```python
from build123d import *

# Parameters (mm, degrees)
F0_W          = 457.2
F0_H          = 254
F1_DEPTH      = 12.7
F3_R          = 15.875
F4_DEPTH      = 25.4
F4_DEPTH_BACK = 25.4
F6_DEPTH      = 127
F6_DEPTH_BACK = 127


with BuildPart() as f1:
    # F0 (on Front) → F1 (new body)
    with BuildSketch(Plane.XZ):
        with Locations((228.6, -127)):
            Rectangle(F0_W, F0_H)
    extrude(amount=F1_DEPTH)

    # F3 (on offset) → F4 (join, two sides)
    with BuildSketch(Plane.XY.offset(-127)) as f4_sk:
        with BuildLine():
            ThreePointArc((25.4, 25.4), (17.9605122421, 7.4394877579), (0, 0))
            Line((0, 0), (25.4, 0))
            Line((25.4, 0), (50.8, 0))
            Line((50.8, 0), (76.2, 0))
            Line((76.2, 0), (101.6, 0))
            ThreePointArc((101.6, 0), (83.6394877579, 7.4394877579), (76.2, 25.4))
            ThreePointArc((76.2, 25.4), (50.8, 50.8), (25.4, 25.4))
        make_face()
        with Locations((50.8, 25.4)):
            Circle(F3_R, mode=Mode.SUBTRACT)
        with BuildLine():
            Line((425.45, 0), (450.85, 0))
            ThreePointArc((450.85, 0), (432.8894877579, 7.4394877579), (425.45, 25.4))
            ThreePointArc((425.45, 25.4), (400.05, 50.8), (374.65, 25.4))
            ThreePointArc((374.65, 25.4), (367.2105122421, 7.4394877579), (349.25, 0))
            Line((349.25, 0), (374.65, 0))
            Line((374.65, 0), (400.05, 0))
            Line((400.05, 0), (425.45, 0))
        make_face()
        with Locations((400.05, 25.4)):
            Circle(F3_R, mode=Mode.SUBTRACT)
    extrude(amount=F4_DEPTH)
    extrude(f4_sk.sketch, amount=-F4_DEPTH_BACK)

    # F5 (on offset) → F6 (cut, two sides)
    with BuildSketch(Plane.XY.offset(-127)) as f6_sk:
        Polygon((25.4, -43.3393605053), (25.4, 0), (25.4, 52.3727163672), (-28.9033520967, 52.3727163672), (-28.9033520967, -43.3393605053), align=None)
        Polygon((425.45, 52.3727163672), (425.45, 0), (425.45, -43.3393605053), (479.7533520967, -43.3393605053), (479.7533520967, 52.3727163672), align=None)
    extrude(amount=-F6_DEPTH, mode=Mode.SUBTRACT)
    extrude(f6_sk.sketch, amount=F6_DEPTH_BACK, mode=Mode.SUBTRACT)


solid = f1.part
```
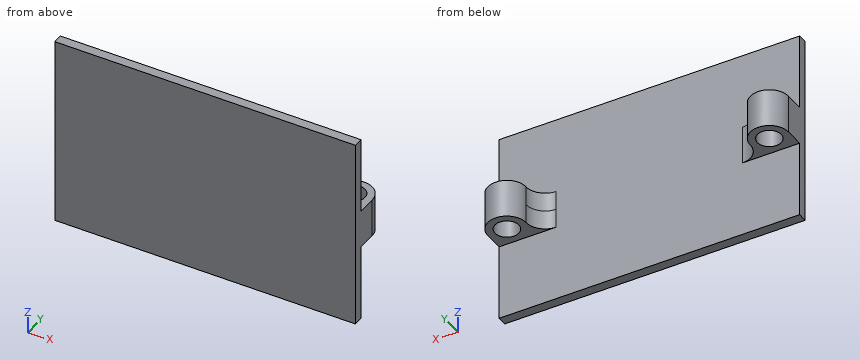
The listing builds one solid part. Answer for the finished solid, in the listing's coordinates (mm). Coordinates: 2 decimals unless noted, no trailing zeros. Loops run counter-clockwise (first coordinate to the right, second up) from the corner with the lowest first, then second, coordinate; pieces in that order, holes last. Notation, with made-up numbers: (80.5, 55.25) -> (121.5, 55.25) arc R10 cw to (121.5, 74.25) -> close; hole circle Ø6 at (44, 60.25). An arc over 180 degrees is marked (long way). Use one line per item in the form item = value. Start each with the question number.
Item 1: The part is cut by section B-B on z = -139.5. Determine the outline of the cut face in (x, y) (3 decimals), then the cut area to 3 significant figures.
Item 2: The part is cut by section D-D on x = 172. Determine the outline of the cut face in (y, z), then the cut area to 3 significant figures.
Item 3: The part is cut by section A-A on x = 400.05. Determine the outline of the cut face in (y, z) (3 decimals), then the cut area to 3 significant figures.
Item 4: The part is cut by section C-C on y = 5.5. Determine the outline of the cut face in (x, z).
Item 5: Flat-ended cylindrical pins translate along their axes: pin 1 Ø12 at (x, y) = (70.5, 27.5) entering from -Z; pin 2 Ø19 at (x, y) = (400.05, 25.4) entering from -Z (3 decimals). Find the tip coordinate at first contact, or state that the pin passes through.
Item 6: Consider L1, parallel to X at y = 25, z = -110; L2, parallel to Y at x = 50.8, z = -116 (3 decimals); L3, parallel to Y at x = 243.5, z = -191. Determine where each line is inside the solid, lowest interval first. Write a range as [from, to].
Answer key:
q1.outline = (25.4, -12.7) -> (425.45, -12.7) -> (425.45, 25.4) arc R25.4 ccw to (374.65, 25.4) arc R25.4 cw to (349.25, 0) -> (101.6, 0) arc R25.4 cw to (76.2, 25.4) arc R25.4 ccw to (25.4, 25.4) -> close; hole circle Ø31.75 at (50.8, 25.4); hole circle Ø31.75 at (400.05, 25.4)
q1.area = 8,380 mm2
q2.outline = (-12.7, -254) -> (0, -254) -> (0, 0) -> (-12.7, 0) -> close
q2.area = 3,230 mm2
q3.outline = (-12.7, -254) -> (0, -254) -> (0, -152.4) -> (9.525, -152.4) -> (9.525, -101.6) -> (0, -101.6) -> (0, 0) -> (-12.7, 0) -> close; (41.275, -152.4) -> (50.8, -152.4) -> (50.8, -101.6) -> (41.275, -101.6) -> close
q3.area = 4,190 mm2
q4.outline = (25.4, -152.4) -> (85.82, -152.4) -> (85.82, -101.6) -> (25.4, -101.6) -> close; (365.03, -152.4) -> (425.45, -152.4) -> (425.45, -101.6) -> (365.03, -101.6) -> close
q5.pin_1 = -152.4
q5.pin_2 = through
q6.L1 = [25.4, 34.93], [66.67, 76.2], [374.65, 384.18], [415.92, 425.45]
q6.L2 = [-12.7, 9.525], [41.275, 50.8]
q6.L3 = [-12.7, 0]
